```python
from build123d import *

# Parameters (mm, degrees)
F1_DEPTH  = 10
F0_R      = 39
F2_DEPTH  = 2
F4_DEPTH  = 3
F5_W      = 20
F5_H      = 4
F6_DEPTH  = 2
F7_W      = 20
F7_H      = 4
F8_DEPTH  = 2
F9_W      = 2
F9_H      = 10
F10_DEPTH = 11.5
F12_DEPTH = 2
F13_R     = 1.25
F14_DEPTH = 3
F16_R     = 1.25
F17_DEPTH = 2
F18_DEPTH = 5


# Not quite as in the source:
# - a feature names something its author has since deleted; it is built from what else it names


with BuildPart() as f1:
    # F0 (on Top) → F1 (new body)
    with BuildSketch(Plane.XY):
        with BuildLine():
            ThreePointArc((69.5, 44.75), (68.0355339059, 48.2855339059), (64.5, 49.75))
            Line((64.5, 49.75), (-64.5, 49.75))
            ThreePointArc((-64.5, 49.75), (-68.0355339059, 48.2855339059), (-69.5, 44.75))
            Line((-69.5, 44.75), (-69.5, -44.75))
            ThreePointArc((-69.5, -44.75), (-68.0355339059, -48.2855339059), (-64.5, -49.75))
            Line((-64.5, -49.75), (64.5, -49.75))
            ThreePointArc((64.5, -49.75), (68.0355339059, -48.2855339059), (69.5, -44.75))
            Line((69.5, -44.75), (69.5, 44.75))
        make_face()
        with BuildLine():
            Line((-62.5, 47.75), (62.5, 47.75))
            ThreePointArc((62.5, 47.75), (66.0355339059, 46.2855339059), (67.5, 42.75))
            Line((67.5, 42.75), (67.5, -42.75))
            ThreePointArc((67.5, -42.75), (66.0355339059, -46.2855339059), (62.5, -47.75))
            Line((62.5, -47.75), (-62.5, -47.75))
            ThreePointArc((-62.5, -47.75), (-66.0355339059, -46.2855339059), (-67.5, -42.75))
            Line((-67.5, -42.75), (-67.5, 42.75))
            ThreePointArc((-67.5, 42.75), (-66.0355339059, 46.2855339059), (-62.5, 47.75))
        make_face(mode=Mode.SUBTRACT)
    extrude(amount=F1_DEPTH)

    # F0 (on Top) → F2 (join)
    with BuildSketch(Plane.XY):
        with BuildLine():
            ThreePointArc((67.5, 42.75), (66.0355339059, 46.2855339059), (62.5, 47.75))
            Line((62.5, 47.75), (-62.5, 47.75))
            ThreePointArc((-62.5, 47.75), (-66.0355339059, 46.2855339059), (-67.5, 42.75))
            Line((-67.5, 42.75), (-67.5, -42.75))
            ThreePointArc((-67.5, -42.75), (-66.0355339059, -46.2855339059), (-62.5, -47.75))
            Line((-62.5, -47.75), (62.5, -47.75))
            ThreePointArc((62.5, -47.75), (66.0355339059, -46.2855339059), (67.5, -42.75))
            Line((67.5, -42.75), (67.5, 42.75))
        make_face()
        Circle(F0_R, mode=Mode.SUBTRACT)
    extrude(amount=F2_DEPTH)

    # F3 (on face) → F4 (join)
    with BuildSketch(Plane.XY.offset(10)):
        with BuildLine():
            Line((20, -49.75), (-20, -49.75))
            Line((-20, -49.75), (-20, -59.75))
            ThreePointArc((-20, -59.75), (-18.5355339059, -63.2855339059), (-15, -64.75))
            Line((-15, -64.75), (15, -64.75))
            ThreePointArc((15, -64.75), (18.5355339059, -63.2855339059), (20, -59.75))
            Line((20, -59.75), (20, -49.75))
        make_face()
    extrude(amount=-F4_DEPTH)

    # F5 (on face) → F6 (cut, through all)
    with BuildSketch(Plane.YZ.offset(-67.5)):
        with Locations((0, 4)):
            Rectangle(F5_W, F5_H)
    extrude(amount=-F6_DEPTH, mode=Mode.SUBTRACT)

    # F7 (on face) → F8 (cut, through all)
    with BuildSketch(Plane(origin=(67.5, 0, 0), x_dir=(0, -1, 0), z_dir=(-1, 0, 0))):
        with Locations((0, 4)):
            Rectangle(F7_W, F7_H)
    extrude(amount=-F8_DEPTH, mode=Mode.SUBTRACT)

    # F9 (on face) → F10 (join)
    with BuildSketch(Plane(origin=(0, 49.75, 0), x_dir=(-1, 0, 0), z_dir=(0, 1, 0))):
        with Locations((51, 5)):
            Rectangle(F9_W, F9_H)
    extrude(amount=F10_DEPTH)

    # F11 (on face) → F12 (join)
    with BuildSketch(Plane(origin=(-52, 0, 0), x_dir=(0, -1, 0), z_dir=(-1, 0, 0))):
        with BuildLine():
            Line((-61.25, 0), (-61.25, 10))
            ThreePointArc((-61.25, 10), (-66.25, 5), (-61.25, 0))
        make_face()
    extrude(amount=-F12_DEPTH)

    # F13 (on face) → F14 (join)
    with BuildSketch(Plane.YZ.offset(-50)):
        with Locations((61.25, 5)):
            Circle(F13_R)
    extrude(amount=F14_DEPTH)

    # F16 (on offset) → F17 (join)
    with BuildSketch(Plane.YZ.offset(52)):
        with BuildLine():
            Line((61.25, 10), (49.75, 10))
            Line((49.75, 10), (49.75, 0))
            Line((49.75, 0), (61.25, 0))
            ThreePointArc((61.25, 0), (66.25, 5), (61.25, 10))
        make_face()
        with Locations((61.25, 5)):
            Circle(F16_R, mode=Mode.SUBTRACT)
    extrude(amount=-F17_DEPTH)

    # F16 (on offset) → F18 (join)
    with BuildSketch(Plane.YZ.offset(52)):
        with Locations((61.25, 5)):
            Circle(F16_R)
    extrude(amount=-F18_DEPTH)


solid = f1.part
```
Can you work these out from the model? Positions are in its coordinate system, mm. A direction names the side the tool comes from. Give positions to 0.01 mm unless a question says otherwise; leave off trailing zeros. Loops run counter-clockwise (first coordinate to the right, second up) from the corner with the lowest first, then second, coordinate; pieces in that order, holes last. Notation, with made-up numbers: M 82.25,78.25 L 102.25,78.25 A10 ccw 102.25,87.25 Z; hole C -29.5,33 d5. An arc over 180 degrees is marked long. One line per question, with ' | ' between items. Start each with the question number.
Q1. If we section it at A-A (y = 54): Please give me the cut outline in (x, z), plus the area to 3 significant figures.
Q2. If we section it at B-B (x = 0): Please give me the cut outline in (y, z).
Q3. If we section it at D-D (x = -59.5): Please give me the cut outline in (y, z), plus the area to 3 significant figures.
Q4. If we mould it in two halves opening along X, with no side actions, what happens to faces 6 (the cylindrical face through (-68, 48.32, 4.93)), 7 (the cylindrical face through (-5.077, 38.668, 0.986)), 8 (the flat face through (-1, -49.75, 5))? For each: +X half, -X half, draft (parallel to the pull), parting line (faces both ways), or undercut.
Q5. If we section it at C-C (y = 0): Please give me the cut outline in (x, z).
Q6. For pin 1 Ø1.5 at (y, z) = (-57, 9) entering from +X; pin 2 Ø3 at (x, z) = (6.5, 5) entering from +Y; pin 3 Ø3 at (x, z) = (-19.5, 3) entering from -Y, each with a flat end and sliding along its axis, tell me the tip position at first contact or that it passes through.
Q7. For faces 1 (the flat face through (0, -57, 7)), 2 (the flat face through (1, -47.75, 6)), 3 (the flat face through (20, -55, 9)), 4 (the flat face through (0, -48, 10)), 5 (the flat face through (52, 58, 5)), which set-ups out of +Z, -Z, +X, -X, +Y, -Y let a thin tool reach every point of the face, with its end or its side?
Q8. If I drill on line 1 (Y direction, x = 33, z = 3); line 2 (Y direction, x = 0, z = 0.75); line 3 (Z direction, x = -42.5, y = 41), over which ranges is the centre line in solid material (lowest first)? Write a range as from..to.
Computed:
1) outline: M -52,0 L -50,0 L -50,10 L -52,10 Z; M 50,0 L 52,0 L 52,10 L 50,10 Z | area: 40.0 mm²
2) outline: M -64.75,7 L -49.75,7 L -49.75,0 L -39,0 L -39,2 L -47.75,2 L -47.75,10 L -64.75,10 Z; M 39,0 L 49.75,0 L 49.75,10 L 47.75,10 L 47.75,2 L 39,2 Z
3) outline: M -49.75,0 L 49.75,0 L 49.75,10 L 47.75,10 L 47.75,2 L -47.75,2 L -47.75,10 L -49.75,10 Z | area: 231 mm²
4) face 6: -X half | face 7: undercut | face 8: draft
5) outline: M -69.5,0 L -39,0 L -39,2 L -69.5,2 Z; M -69.5,6 L -67.5,6 L -67.5,10 L -69.5,10 Z; M 39,0 L 69.5,0 L 69.5,2 L 39,2 Z; M 67.5,6 L 69.5,6 L 69.5,10 L 67.5,10 Z
6) pin 1: stops at x = 20 | pin 2: stops at y = 49.75 | pin 3: stops at y = -49.75
7) face 1: -Z, +X, -X, -Y | face 2: +Z | face 3: +Z, -Z, +X, -Y | face 4: +Z, +X, -X, +Y, -Y | face 5: +Z, -Z, +X, +Y
8) line 1: y = -49.75..-47.75, 47.75..49.75 | line 2: y = -49.75..-39, 39..49.75 | line 3: z = 0..2
